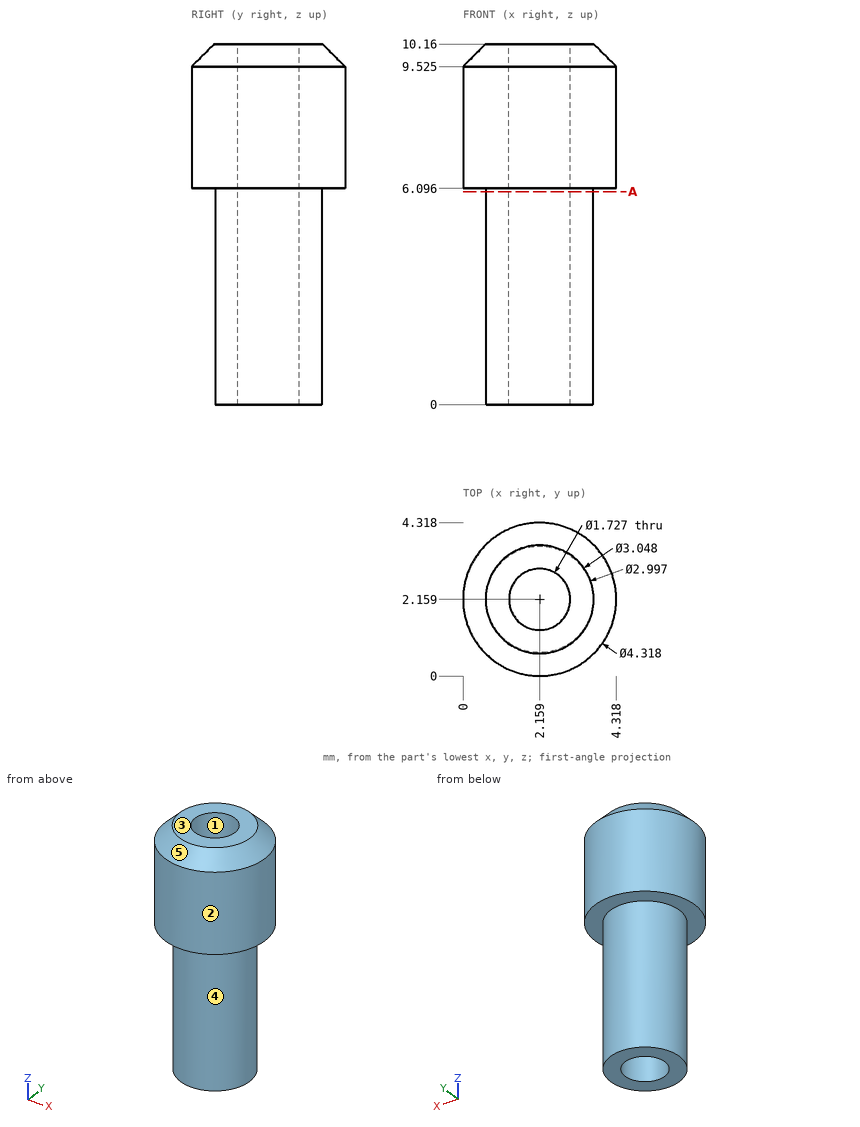
Verification items for this drawing (mm, ordinates from the low corner). A direction names the side the tool comes from. Coordinates: 2 decimals unless noted, no trailing zeros. Write each loop counter-clockwise with the first axis right and the second up, starting at its lowest first coordinate (ties: lowest second). Pieces come first, ordered by that corner, then holes. Notation, with made-up numbers: (87.25, 85.5) - (116.25, 85.5) arc R34 cw to (116.25, 120.5) - close; hole circle Ø5 at (-7, 62.5). An arc over 180 degrees is marked (long way). One line per question, with ' | ' between items.
Item 1: Access from +Z, -Z, +X, -X, +Y, -Y to the whole of each face (thin tool, end or side, straight path). Record for the marked faces 4 and 5.
Determined:
face 4: -Z | face 5: +Z
Item 2: Thickness scan on line 1 (X direction, y = 1.8, z = 6) (1 decimal); line 2 (X direction, y = 2.15, z = 8.75); line 3 (Y direction, x = 2.7, z = 5.75) (1 decimal). Record the ranges inside material, lowest first. Write a range as [from, to].
Determined:
line 1: x = [0.7, 1.4], [2.9, 3.6] | line 2: x = [0, 1.3], [3.02, 4.32] | line 3: y = [0.8, 1.5], [2.8, 3.6]
Item 3: Mould release check, pull along X, two halves, no side actions. Record for the marked faces 1, 2 and 3: pulls with the +X half, pulls with the -X half, needs draft (parallel to the pull), parting line crosses it, or undercut.
Determined:
face 1: undercut | face 2: parting line crosses it | face 3: needs draft
Item 4: Sectioned sample at A-A on z = 6. Record the boundary of the cut face in (x, y).
Determined:
outline: circle Ø3 at (2.16, 2.16); hole circle Ø1.73 at (2.16, 2.16)
